from build123d import *
from build123d.topology import SkipClean

# Parameters (mm, degrees)
SKETCH1_W              = 49
SKETCH1_H              = 50
BOSS_EXTRUDE1_DEPTH    = 3
SKETCH2_W              = 5
SKETCH2_H              = 50
BOSS_EXTRUDE2_DEPTH    = 55
SKETCH3_OUTSIDE_W      = 78.182
SKETCH3_OUTSIDE_H      = 70.182
SKETCH3_OUTSIDE_R      = 4
CUT_EXTRUDE1_DEPTH     = 80.937475567
SKETCH4_R              = 7.5
SKETCH4_R_2            = 5
BOSS_EXTRUDE3_DEPTH    = 15
SKETCH5_R              = 10
SKETCH5_R_2            = 4
BOSS_EXTRUDE4_DEPTH    = 8
CUT_EXTRUDE2_START     = -5
CUT_EXTRUDE2_OUTLINE_R = 1.5
CUT_EXTRUDE2_DEPTH     = 5
SKETCH7_W              = 80
SKETCH7_H              = 50
BOSS_EXTRUDE5_DEPTH    = 3


# Read off the part's stored shape, not the designer's step: Cut-Extrude2
with BuildPart() as part:
    # Sketch1 → Boss-Extrude1 (new body)
    with BuildSketch(Plane.XY):
        Rectangle(SKETCH1_W, SKETCH1_H)
    extrude(amount=BOSS_EXTRUDE1_DEPTH)

    # Sketch2 → Boss-Extrude2 (add)
    with BuildSketch(Plane.XY.offset(3)):
        with Locations((-22, 0)):
            Rectangle(SKETCH2_W, SKETCH2_H)
        with Locations((22, 0)):
            Rectangle(SKETCH2_W, SKETCH2_H)
    extrude(amount=BOSS_EXTRUDE2_DEPTH)

    # Sketch3 outside → Cut-Extrude1 (cut, through all)
    # profile 1 of 2: a face of its own
    with BuildSketch(Plane.ZY.offset(24.5)):
        with Locations((29, 0)):
            Rectangle(SKETCH3_OUTSIDE_W, SKETCH3_OUTSIDE_H)
        with BuildLine():
            Line((0, 25), (0, -25))
            Line((0, -25), (33, -25))
            ThreePointArc((33, -25), (58, 0), (33, 25))
            Line((33, 25), (0, 25))
        make_face(mode=Mode.SUBTRACT)
    # profile 2 of 2: a face of its own
    with BuildSketch(Plane.ZY.offset(24.5)):
        with Locations((33, 0)):
            Circle(SKETCH3_OUTSIDE_R)
    extrude(amount=-CUT_EXTRUDE1_DEPTH, mode=Mode.SUBTRACT)

    # Sketch4 → Boss-Extrude3 (add)
    with BuildSketch(Plane.XY.offset(3)):
        with Locations((0, 10)):
            Circle(SKETCH4_R)
        with Locations((0, 10)):
            Circle(SKETCH4_R_2, mode=Mode.SUBTRACT)
    extrude(amount=BOSS_EXTRUDE3_DEPTH)

    # Sketch5 → Boss-Extrude4 (add)
    with SkipClean():  # the faces are left unmerged after this step: merging them gives an invalid solid
        with BuildSketch(Plane(origin=(24.5, 0, 0), x_dir=(0, 0, -1), z_dir=(1, 0, 0))):
            with Locations(Location((-33, 0, 0), (0, 0, 270))):
                Circle(SKETCH5_R)
            with Locations(Location((-33, 0, 0), (0, 0, 90))):
                Circle(SKETCH5_R_2, mode=Mode.SUBTRACT)
        extrude(amount=BOSS_EXTRUDE4_DEPTH)

    # Cut-Extrude2 outline → Cut-Extrude2 (cut)
    with SkipClean():  # the faces are left unmerged after this step: merging them gives an invalid solid
        with BuildSketch(Plane(origin=(24.5, 0, 0), x_dir=(0, 0, -1), z_dir=(1, 0, 0)).offset(CUT_EXTRUDE2_START)):
            with Locations((-42.744235689, 10.052356482)):
                Circle(CUT_EXTRUDE2_OUTLINE_R)
            with Locations((-22.947643518, 9.744235689)):
                Circle(CUT_EXTRUDE2_OUTLINE_R)
            with Locations((-23.255764311, -10.052356482)):
                Circle(CUT_EXTRUDE2_OUTLINE_R)
            with Locations((-43.052356482, -9.744235689)):
                Circle(CUT_EXTRUDE2_OUTLINE_R)
        extrude(amount=CUT_EXTRUDE2_DEPTH, mode=Mode.SUBTRACT)

    # Sketch7 → Boss-Extrude5 (add)
    with SkipClean():  # the faces are left unmerged after this step: merging them gives an invalid solid
        with BuildSketch(Plane(origin=(0, 0, 0), x_dir=(-1, 0, 0), z_dir=(0, 0, -1))):
            Rectangle(SKETCH7_W, SKETCH7_H)
        extrude(amount=-BOSS_EXTRUDE5_DEPTH)


solid = part.part
Input: part model. Units: mm. Frame: model coordinates. A direction names the side the tool comes from. Coordinates: 2 decimals unless noted, no trailing zeros. Loops run counter-clockwise (first coordinate to the right, second up) from the corner with the lowest first, then second, coordinate; pieces in that order, holes last. Notation, with made-up numbers: (33, -36) - (73, -36) arc R20 ccw to (73, -3) - close; hole circle Ø6 at (-34.75, 9). An arc over 180 degrees is marked (long way). Answer in a Markdown table with one row per item. Add a question column.
Item 1: Section query C-C on z = 53.5. Return the cut outline in (x, y).
Item 2: Line query: line 1 along X through (y, z) = (-4, 37.5); line 2 along X through (y, z) = (6.5, 52.5); line 3 along X through (y, z) = (5.5, 7). Output: solid intervals per line, ascending. Write a range as [from, to].
Item 3: Access query for faces 4 (the flat face through (0, 10, 3)), 5 (the flat face through (-24.5, 0, 24)), 6 (the flat face through (32, 0, 3)). Directions: +Z, -Z, +X, -X, +Y, -Y. A direction counts if a zero-diameter tool reaches every point of the face in a straight line with its end or side. Return the directions, or none.
Item 4: Contact query for flat-ended pins moving along their axis: P1, Ø10.5, axis at y = 0, z = 33, coming from the +X side; P2, Ø3, axis at x = -1.5, y = 9, coming from the +Z side; P3, Ø3, axis at y = -18.5, z = 16.5, coming from the -X side; P4, Ø3, axis at x = 11, y = 20, coming from the -Z side. Output: stop coordinate, or through.
Item 5: Section query B-B on x = 0. Return the cut outline in (y, z), then the cut area to 3 significant figures.
Item 6: Section query A-A on z = 19. Return the cut outline in (x, y), then the cut area to 3 significant figures.
Item 7: Section query D-D on x = 10.5. Return the cut outline in (y, z).
Item 8: Mould query, pull axis X, two halves, no side actions, for faces 1 (the cylindrical face through (21.965, -0.55, 57.994)), 2 (the flat face through (2, 5, 18)), 3 (the flat face through (-40, 0, 1)). Classes: released by +X, released by -X, zero draft, split by the parting line, or undercut.
Recorded:
| question | item | result |
|---|---|---|
| 1 | outline | (-24.5, -14.31) - (-19.5, -14.31) - (-19.5, 14.31) - (-24.5, 14.31) - close; (19.5, -14.31) - (24.5, -14.31) - (24.5, 14.31) - (19.5, 14.31) - close |
| 2 | line 1 | [-24.5, -19.5], [19.5, 32.5] |
| 2 | line 2 | [-24.5, -19.5], [19.5, 24.5] |
| 2 | line 3 | [-24.5, -19.5], [-6, -2.18], [2.18, 6], [19.5, 24.5] |
| 3 | face 4 | +Z |
| 3 | face 5 | +Z, -X, +Y, -Y |
| 3 | face 6 | +X, +Y, -Y |
| 4 | P1 | x = 32.5 |
| 4 | P2 | z = 3 |
| 4 | P3 | x = -24.5 |
| 4 | P4 | z = 0 |
| 5 | outline | (-25, 0) - (25, 0) - (25, 3) - (17.5, 3) - (17.5, 18) - (15, 18) - (15, 3) - (5, 3) - (5, 18) - (2.5, 18) - (2.5, 3) - (-25, 3) - close |
| 5 | area | 225 mm^2 |
| 6 | outline | (-24.5, -25) - (-19.5, -25) - (-19.5, 25) - (-24.5, 25) - close; (19.5, -25) - (24.5, -25) - (24.5, 25) - (19.5, 25) - close |
| 6 | area | 500 mm^2 |
| 7 | outline | (-25, 0) - (25, 0) - (25, 3) - (-25, 3) - close |
| 8 | face 1 | zero draft |
| 8 | face 2 | undercut |
| 8 | face 3 | released by -X |
